```python
from build123d import *

# Parameters (mm, degrees)
F0_R     = 24.5
F0_R_2   = 22.5
F1_DEPTH = 60
F4_W     = 21.917041
F4_H     = 35.913566
F5_DEPTH = 25


with BuildPart() as f1:
    # F0 (on Top) → F1 (new body)
    with BuildSketch(Plane.XY):
        Circle(F0_R)
        Circle(F0_R_2, mode=Mode.SUBTRACT)
    extrude(amount=F1_DEPTH)

    # F2 (on Front) → F3 (revolve)
    with BuildSketch(Plane.XZ):
        Polygon((23.440696, 11.506858), (22.541139, 11.506858), (19.177632, 0), (23.440696, 0), align=None)
    revolve(axis=Axis((0, 0, 8.668173), (0, 0, -1)))

    # F4 (on Front) → F5 (cut)
    with BuildSketch(Plane.XZ):
        with Locations((0.000676, 13.722296)):
            Rectangle(F4_W, F4_H)
    extrude(amount=F5_DEPTH, mode=Mode.SUBTRACT)


solid = f1.part
```
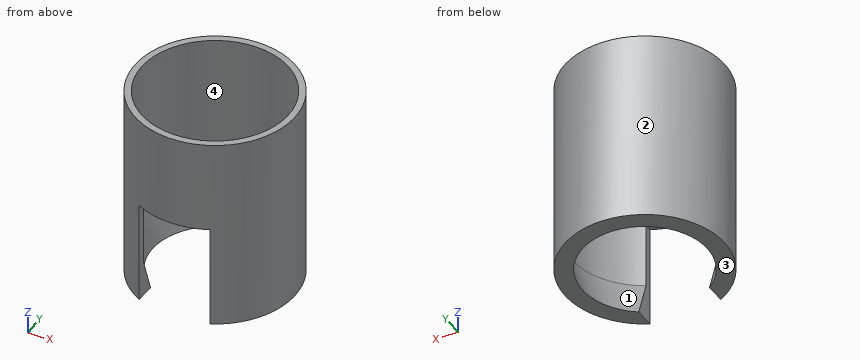
Design review of the part built by this model. Coordinates are the model's own, in mm. Face numbers are marked on the shaded views. Give positions to 0.01 mm unless a question says otherwise; leave off trailing zeros. Order: outer loops, then holes, each group sorted by start corner. A loop starts at its lowest first (then second) coordinate and runs counter-clockwise, first axis right, second up. Notation, with made-up numbers: M 8,82 L 17,82 A29 cw 17,105 Z; hole C -35,-37.75 d7. An arc over 180 degrees is marked long. One line per question, with ' | ' between items. Start each with the question number.
Q1. We need section A-A (x = 0). Write out the cut boundary in (y, z), plus the area to 3 significant figures.
Q2. We need section C-C (z = 55). Write out the cut boundary in (x, y).
Q3. For pin 1 Ø1.5 at (y, z) = (1.5, 14) entering from +X; pin 2 Ø7 at (y, z) = (-18, 19.5) entering from -X; pin 3 Ø1.5 at (x, y) = (-3.5, -21.5) entering from -Z, all flat-tipped, find the tip position at first contact; note any pin that passes through.
Q4. For L1, parallel to Y at x = 0, z = 42; L2, parallel to Y at x = 0, z = 23, list the stretches that pass through material, from the lowest coordinate up. Write a range as [from, to].
Q5. The part is to be moulded in two halves that separate along Y. For the marked faces 1, 2, 3 and 4, say which applies: +Y half, -Y half, draft (parallel to the pull), parting line (faces both ways), or undercut.
Q6. We need section B-B (y = 0). Write out the cut boundary in (x, z).
Q7. We need section D-D (z = 13.5). Write out the cut boundary in (x, y).
Returned:
1) outline: M -24.5,31.68 L -22.5,31.68 L -22.5,60 L -24.5,60 Z; M 19.18,0 L 24.5,0 L 24.5,60 L 22.5,60 L 22.5,11.37 Z | area: 196 mm2
2) outline: C 0,0 d49; hole C 0,0 d45
3) pin 1: x = 24.49 | pin 2: x = -19.75 | pin 3: z = 31.68
4) L1: [-24.5, -22.5], [22.5, 24.5] | L2: [22.5, 24.5]
5) face 1: undercut | face 2: parting line | face 3: draft | face 4: undercut
6) outline: M -24.5,0 L -19.18,0 L -22.5,11.37 L -22.5,60 L -24.5,60 Z; M 19.18,0 L 24.5,0 L 24.5,60 L 22.5,60 L 22.5,11.37 Z
7) outline: M -10.96,-21.91 L -10.96,-19.65 A22.5 cw long 10.96,-19.65 L 10.96,-21.91 A24.5 ccw long Z
